from build123d import *

# Parameters (mm, degrees)
SKETCH1_W           = 210.82
SKETCH1_H           = 257.175
SKETCH1_W_2         = 185.42
SKETCH1_H_2         = 231.775
SKETCH1_H_3         = 46.355
BOSS_EXTRUDE1_DEPTH = 3.175
SKETCH3_R           = 2.0955
CUT_EXTRUDE1_DEPTH  = 3.175
BOSS_EXTRUDE2_DEPTH = 3.175
FILLET1_R           = 2.54


with BuildPart() as part:
    # Sketch1 → Boss-Extrude1 (new body)
    with BuildSketch(Plane(origin=(0, 0, 0), x_dir=(1, 0, 0), z_dir=(0, 1, 0))):
        with Locations((92.71, 115.8875)):
            Rectangle(SKETCH1_W, SKETCH1_H)
        with Locations((92.71, 115.8875)):
            Rectangle(SKETCH1_W_2, SKETCH1_H_2, mode=Mode.SUBTRACT)
        with Locations((92.71, 115.8875)):
            Rectangle(SKETCH1_W_2, SKETCH1_H_2)
        with Locations((92.71, 208.5975)):
            Rectangle(SKETCH1_W_2, SKETCH1_H_3)
    extrude(amount=BOSS_EXTRUDE1_DEPTH)

    # Sketch3 → Cut-Extrude1 (cut)
    with BuildSketch(Plane(origin=(0, 3.175, 0), x_dir=(1, 0, 0), z_dir=(0, 1, 0))):
        with BuildLine():
            ThreePointArc((61.244272613, 244.475), (75.743989862, 235.069736233), (92.71, 231.775))
            Line((92.71, 231.775), (92.71, 244.475))
            Line((92.71, 244.475), (61.244272613, 244.475))
        make_face()
        with BuildLine():
            Line((92.71, 244.475), (92.71, 231.775))
            ThreePointArc((92.71, 231.775), (109.676010138, 235.069736233), (124.175727387, 244.475))
            Line((124.175727387, 244.475), (92.71, 244.475))
        make_face()
        with Locations(Location((191.77, 238.125, 0), (0, 0, 270))):
            Circle(SKETCH3_R)
        with Locations(Location((191.77, -6.35, 0), (0, 0, 270))):
            Circle(SKETCH3_R)
        with Locations(Location((-6.35, -6.35, 0), (0, 0, 270))):
            Circle(SKETCH3_R)
        with Locations(Location((-6.35, 238.125, 0), (0, 0, 270))):
            Circle(SKETCH3_R)
    extrude(amount=-CUT_EXTRUDE1_DEPTH, mode=Mode.SUBTRACT)

    # Sketch3_3 → Boss-Extrude2 (add)
    with BuildSketch(Plane(origin=(0, 3.175, 0), x_dir=(1, 0, 0), z_dir=(0, 1, 0))):
        with BuildLine():
            ThreePointArc((138.04, 277.105), (134.430200877, 259.378360759), (124.175727387, 244.475))
            Line((124.175727387, 244.475), (146.685, 244.475))
            Line((146.685, 244.475), (146.685, 301.625))
            Line((146.685, 301.625), (142.4305, 301.625))
            ThreePointArc((142.4305, 301.625), (138.85325774, 300.14325774), (140.335, 303.7205))
            Line((140.335, 303.7205), (140.335, 307.975))
            Line((140.335, 307.975), (125.904156112, 307.975))
            ThreePointArc((125.904156112, 307.975), (134.897083311, 293.68989981), (138.04, 277.105))
        make_face()
        with BuildLine():
            Line((142.4305, 301.625), (146.685, 301.625))
            Line((146.685, 301.625), (146.685, 307.975))
            Line((146.685, 307.975), (140.335, 307.975))
            Line((140.335, 307.975), (140.335, 303.7205))
            ThreePointArc((140.335, 303.7205), (141.81674226, 303.10674226), (142.4305, 301.625))
        make_face()
        with BuildLine():
            Line((38.735, 244.475), (61.244272613, 244.475))
            ThreePointArc((61.244272613, 244.475), (47.396783015, 275.871603687), (59.515843888, 307.975))
            Line((59.515843888, 307.975), (45.085, 307.975))
            Line((45.085, 307.975), (45.085, 303.7205))
            ThreePointArc((45.085, 303.7205), (46.56674226, 303.10674226), (47.1805, 301.625))
            ThreePointArc((47.1805, 301.625), (45.085, 299.5295), (42.9895, 301.625))
            Line((42.9895, 301.625), (38.735, 301.625))
            Line((38.735, 301.625), (38.735, 244.475))
        make_face()
        with BuildLine():
            Line((38.735, 307.975), (38.735, 301.625))
            Line((38.735, 301.625), (42.9895, 301.625))
            ThreePointArc((42.9895, 301.625), (43.60325774, 303.10674226), (45.085, 303.7205))
            Line((45.085, 303.7205), (45.085, 307.975))
            Line((45.085, 307.975), (38.735, 307.975))
        make_face()
    extrude(amount=-BOSS_EXTRUDE2_DEPTH)

    # Fillet1
    fillet1_edges = [part.edges().sort_by_distance(p)[0] for p in [
        (146.685, 1.5875, -307.975),
        (146.685, 1.5875, -244.475),
        (38.735, 1.5875, -307.975),
        (38.735, 1.5875, -244.475),
        (-12.7, 1.5875, -244.475),
        (198.12, 1.5875, -244.475),
        (198.12, 1.5875, 12.7),
        (-12.7, 1.5875, 12.7),
    ]]
    fillet(fillet1_edges, radius=FILLET1_R)


solid = part.part
Part model, mm, in its own coordinate system. Coordinates: 2 decimals unless noted, no trailing zeros. Loops run counter-clockwise (first coordinate to the right, second up) from the corner with the lowest first, then second, coordinate; pieces in that order, holes last. Notation, with made-up numbers: (13, 16) -> (71, 16) arc R20 ccw to (71, 55) -> close; hole circle Ø2 at (64.25, 72.25). An arc over 180 degrees is marked (long way). Use a Markdown table: item, result. Add a question column.
Item 1: Probe probe 1 along Z at (x, y) = (191.77, 2) (1 decimal); probe 2 along X at (y, z) = (0.6, -240); probe 3 along Z at (x, y) = (-1.5, 1.75) (3 decimals). List the from-to ranges inside material, lowest first.
Item 2: Band-saw the part on B-B on x = 153.5. Write the cut outline in (y, z) (3 decimals), plus the area to 3 significant figures.
Item 3: Flat gauge pins, fed straight in: P1, Ø1.6, axis at x = 16, y = 1.5, coming from the -Z side (3 decimals); P2, Ø3.5, axis at x = 191.77, z = -238.125, coming from the -Y side; P3, Ø1.6, axis at y = 2, z = -280.5, coming from the -X side (3 decimals); P4, Ø1.6, axis at y = 1, z = -286.5, coming from the +X side (3 decimals). Where does each tip first touch, or does it go through?
Item 4: Band-saw the part on A-A on y = 1.2. Give the number of separate pieces and of enclosed holes in the cut face, plus the area to 3 significant figures.
Geometry says:
| question | item | result |
|---|---|---|
| 1 | probe 1 | -244.5 to -240.2, -236 to 4.3, 8.4 to 12.7 |
| 1 | probe 2 | -12.7 to -7.29, -5.41 to 66.67, 118.75 to 190.83, 192.71 to 198.12 |
| 1 | probe 3 | -244.475 to 12.7 |
| 2 | outline | (0, -244.475) -> (3.175, -244.475) -> (3.175, 12.7) -> (0, 12.7) -> close |
| 2 | area | 817 mm² |
| 3 | P1 | z = -244.475 |
| 3 | P2 | through |
| 3 | P3 | x = 38.735 |
| 3 | P4 | x = 146.685 |
| 4 | separate pieces | 1 |
| 4 | enclosed holes | 6 |
| 4 | area | 55,200 mm² |
